Build history of the part. All positions in model axes, mm. Face numbers are marked on the shaded views. A direction names the side the tool comes from. Round coordinates to 2 decimals unless told otherwise and drop trailing zeros. Loops run counter-clockwise (first coordinate to the right, second up) from the corner with the lowest first, then second, coordinate; pieces in that order, holes last.
from build123d import *

# Parameters (mm, degrees)
SKETCH_1_R                   = 7.425
EXTRUDE_1_DEPTH              = 3
SKETCH_2_R                   = 7
EXTRUDE_2_DEPTH              = 12
HOLE_WIZARD_M3_1_D           = 3.4
HOLE_WIZARD_M3_1_CBORE_D     = 6.5
HOLE_WIZARD_M3_1_CBORE_DEPTH = 3.4
CHAMFER_1_SIZE               = 1


with BuildPart() as part:
    # 草图1 → 凸台-拉伸1 (new body)
    with BuildSketch(Plane.XY):
        Circle(SKETCH_1_R)
    extrude(amount=EXTRUDE_1_DEPTH)

    # 草图2 → 凸台-拉伸2 (add)
    with BuildSketch(Plane.XY):
        Circle(SKETCH_2_R)
    extrude(amount=EXTRUDE_2_DEPTH)

    # M3 六角凹头螺钉的柱形沉头孔1 (through all)
    with Locations(Plane(origin=(0, 0, 12), x_dir=(-1, 0, 0), z_dir=(0, 0, 1))):
        with Locations((0, 0)):
            CounterBoreHole(HOLE_WIZARD_M3_1_D / 2, HOLE_WIZARD_M3_1_CBORE_D / 2, HOLE_WIZARD_M3_1_CBORE_DEPTH)

    # 倒角1
    chamfer_1_edges = [part.edges().sort_by_distance(p)[0] for p in [
        (-7, 0, 12),
    ]]
    chamfer(chamfer_1_edges, length=CHAMFER_1_SIZE)


solid = part.part
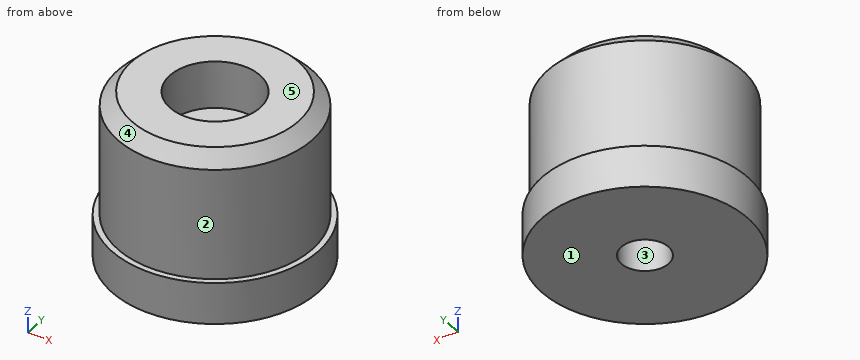
(1) Probe line 1 (Y direction, x = 0, z = 9.8); line 2 (Y direction, x = 0, z = 3.25); line 3 (X direction, y = -4.75, z = 6). List the from-to ranges inside material, lowest first.
Responses:
line 1: y = -7 to -3.25, 3.25 to 7
line 2: y = -7 to -1.7, 1.7 to 7
line 3: x = -5.14 to 5.14
(2) Slice it at C-C on z = 7. List the corners of the cut face in (x, y).
Responses:
outline: circle Ø14 at (0, 0); hole circle Ø3.4 at (0, 0)
(3) Pin check, flat tips, straight feed: P1, Ø4, axis at x = 4.5, z = 9, coming from the -Y side; P2, Ø2, axis at y = -4, z = 8.5, coming from the -X side; P3, Ø2, axis at x = 0, y = 0, coming from the +Z side; P4, Ø6, axis at x = -4, z = 9, coming from the -Y side. Stop position of each tip, or through.
Responses:
P1: stops at y = -6.54
P2: stops at x = -6.32
P3: passes through
P4: stops at y = -6.93
(4) Pull direction X, two halves, no side cores. Call the marked faces 3, 4 and 5: +X half, -X half, draft (parallel to the pull), parting line (faces both ways), or undercut.
Responses:
face 3: undercut
face 4: parting line
face 5: draft
(5) Which spindle directions (+Z, -Z, +X, -X, +Y, -Y) get a long thin tool onto all of the face, cutting with end or side? Do the marked faces 1 and 2. Say none if no direction does.
Responses:
face 1: -Z, +X, -X, +Y, -Y
face 2: +Z
(6) Slice it at D-D on z = 9. List the corners of the cut face in (x, y), plus the area to 3 significant figures.
Responses:
outline: circle Ø14 at (0, 0); hole circle Ø6.5 at (0, 0)
area: 121 mm2
(7) Slice it at A-A on y = 0. List the corners of the cut face in (x, z) (3 decimals).
Responses:
outline: (-7.425, 0) - (-1.7, 0) - (-1.7, 8.6) - (-3.25, 8.6) - (-3.25, 12) - (-6, 12) - (-7, 11) - (-7, 3) - (-7.425, 3) - close; (1.7, 0) - (7.425, 0) - (7.425, 3) - (7, 3) - (7, 11) - (6, 12) - (3.25, 12) - (3.25, 8.6) - (1.7, 8.6) - close
